The model under review builds one solid part; all positions refer to its coordinate system, in mm. A direction names the side the tool comes from. Round coordinates to 2 decimals unless told otherwise and drop trailing zeros. Write each loop counter-clockwise with the first axis right and the second up, starting at its lowest first coordinate (ties: lowest second). Pieces come first, ordered by that corner, then holes. Notation, with made-up numbers: (5, 50.5) - (31, 50.5) arc R24 ccw to (31, 76.5) - close; hole circle Ø6 at (78.5, -32.5). An arc over 180 degrees is marked (long way). Return JSON: item names as keys, results as strings.
from build123d import *

# Parameters (mm, degrees)
ESBO_O7_W                = 40
ESBO_O7_H                = 35
CORTE_EXTRUS_O3_DEPTH    = 20
ESBO_O8_W                = 40
ESBO_O8_H                = 35
RESSALTO_EXTRUS_O1_DEPTH = 60
ESBO_O9_R                = 15
CORTE_EXTRUS_O4_DEPTH    = 30
ESBO_O10_W               = 60
ESBO_O10_H               = 42.668623852
CORTE_EXTRUS_O6_DEPTH    = 5
ESBO_O12_W               = 50
ESBO_O12_H               = 21.334311926
RESSALTO_EXTRUS_O3_DEPTH = 5
ESBO_O13_W               = 60
ESBO_O13_H               = 42.668623852
CORTE_EXTRUS_O8_DEPTH    = 5
ESBO_O14_W               = 50
ESBO_O14_H               = 21.334311926
RESSALTO_EXTRUS_O4_DEPTH = 5
ESBO_O15_W               = 17.17613937
ESBO_O15_H               = 45.233285306
CORTE_EXTRUS_O9_DEPTH    = 5
ESBO_O16_W               = 17.17613937
ESBO_O16_H               = 40
RESSALTO_EXTRUS_O5_DEPTH = 5
ESBO_O17_R               = 2.5
CORTE_EXTRUS_O10_DEPTH   = 10
ESBO_O21_R               = 2.5
CORTE_EXTRUS_O11_DEPTH   = 519.156686831


with BuildPart() as part:
    # Esbo_o2 → Loft1 section 0
    with BuildSketch(Plane.XY, mode=Mode.PRIVATE) as loft1_s0:
        with BuildLine():
            Line((-10.863095238, 0), (204.136904762, 0))
            Line((204.136904762, 0), (77.102021041, 179.616642653))
            Line((77.102021041, 179.616642653), (-10.863095238, 0))
        make_face()
    loft([Vertex(77.102021041, 179.616642653, -400), loft1_s0.sketch])

    # Esbo_o7 → Corte-extrus_o3 (cut)
    with BuildSketch(Plane(origin=(77.102021041, 179.616642653, -400), x_dir=(1, 0, 0), z_dir=(0, 0, 1))):
        Rectangle(ESBO_O7_W, ESBO_O7_H)
    extrude(amount=CORTE_EXTRUS_O3_DEPTH, mode=Mode.SUBTRACT)

    # Esbo_o8 → Ressalto-extrus_o1 (add)
    with BuildSketch(Plane(origin=(0, 0, -380), x_dir=(-1, 0, 0), z_dir=(0, 0, -1))):
        with Locations((-77.5, 174.5)):
            Rectangle(ESBO_O8_W, ESBO_O8_H)
    extrude(amount=RESSALTO_EXTRUS_O1_DEPTH)

    # Esbo_o9 → Corte-extrus_o4 (cut)
    with BuildSketch(Plane(origin=(0, 192, 0), x_dir=(1, 0, 0), z_dir=(0, 1, 0))):
        with Locations(Location((77.5, 410, 0), (0, 0, 270))):
            Circle(ESBO_O9_R)
    extrude(amount=-CORTE_EXTRUS_O4_DEPTH, mode=Mode.SUBTRACT)

    # Esbo_o10 → Corte-extrus_o6 (cut)
    with BuildSketch(Plane.XY):
        with Locations((-10.863095238, 0)):
            Rectangle(ESBO_O10_W, ESBO_O10_H)
    extrude(amount=-CORTE_EXTRUS_O6_DEPTH, mode=Mode.SUBTRACT)

    # Esbo_o12 → Ressalto-extrus_o3 (add)
    with BuildSketch(Plane.XY.offset(-5)):
        with Locations((-5.863095238, 10.667155963)):
            Rectangle(ESBO_O12_W, ESBO_O12_H)
    extrude(amount=RESSALTO_EXTRUS_O3_DEPTH)

    # Esbo_o13 → Corte-extrus_o8 (cut)
    with BuildSketch(Plane.XY):
        with Locations((204.136904762, 0)):
            Rectangle(ESBO_O13_W, ESBO_O13_H)
    extrude(amount=-CORTE_EXTRUS_O8_DEPTH, mode=Mode.SUBTRACT)

    # Esbo_o14 → Ressalto-extrus_o4 (add)
    with BuildSketch(Plane.XY.offset(-5)):
        with Locations((199.136904762, 10.667155963)):
            Rectangle(ESBO_O14_W, ESBO_O14_H)
    extrude(amount=RESSALTO_EXTRUS_O4_DEPTH)

    # Esbo_o15 → Corte-extrus_o9 (cut)
    with BuildSketch(Plane.XY):
        with Locations((77.102021041, 179.616642653)):
            Rectangle(ESBO_O15_W, ESBO_O15_H)
    extrude(amount=-CORTE_EXTRUS_O9_DEPTH, mode=Mode.SUBTRACT)

    # Esbo_o16 → Ressalto-extrus_o5 (add)
    with BuildSketch(Plane.XY.offset(-5)):
        with Locations((77.102021041, 177)):
            Rectangle(ESBO_O16_W, ESBO_O16_H)
    extrude(amount=RESSALTO_EXTRUS_O5_DEPTH)

    # Esbo_o17 → Corte-extrus_o10 (cut)
    with BuildSketch(Plane.XY):
        with Locations((-20.863095238, 11.334311926)):
            Circle(ESBO_O17_R)
        with Locations((214.136904762, 10)):
            Circle(ESBO_O17_R)
        with Locations((77.190090726, 187)):
            Circle(ESBO_O17_R)
    extrude(amount=-CORTE_EXTRUS_O10_DEPTH, mode=Mode.SUBTRACT)

    # Esbo_o20 → Loft de corte2 section 0
    with BuildSketch(Plane.XY, mode=Mode.PRIVATE) as loft_de_corte2_s0:
        with BuildLine():
            Line((4.64946483, 2.5), (184.871981239, 2.5))
            Line((184.871981239, 2.5), (184.871981239, 22.909462338))
            Line((184.871981239, 22.909462338), (88.571698608, 159.069963659))
            Line((88.571698608, 159.069963659), (69.823235581, 159.069963659))
            Line((69.823235581, 159.069963659), (4.64946483, 25.99114348))
            Line((4.64946483, 25.99114348), (4.64946483, 2.5))
        make_face()
    loft([loft_de_corte2_s0.sketch, Vertex(77.102021041, 179.616642653, -400)], mode=Mode.SUBTRACT)

    # Esbo_o21 → Corte-extrus_o11 (cut, through all)
    with BuildSketch(Plane.XZ.offset(-157)):
        with Locations(Location((77.5, -410, 0), (0, 0, 270))):
            Circle(ESBO_O21_R)
    extrude(amount=-CORTE_EXTRUS_O11_DEPTH, mode=Mode.SUBTRACT)


solid = part.part
(1) For faces 1 (the flat face through (91, 192, -403)), 2 (the flat face through (143, 84, 0)), 3 (the flat face through (29.994, 71.049, -139.923)), 4 (the cylindrical face through (71.755, 177.21, -396.144)), list the 3-axis set-ups (+Z, -Z, +X, -X, +Y, -Y) from which the entire face can be reached by the end or side of a thin tool; tool diameter is ignored.
Filled in:
{"face 1": "-Z, +X, -X, +Y", "face 2": "+Z, +X, -X, +Y, -Y", "face 3": "none", "face 4": "+Y"}
(2) Wall thickness on line 1 (X direction, y = 158.55, z = -410); line 2 (X direction, y = 140.5, z = -188); line 3 (Y direction, x = 72, z = -148): over which ranges is each line inside the solid? List them lowest first.
Filled in:
{"line 1": "x = 57.5 to 75, 80 to 97.5", "line 2": "x = 57.95 to 59.42, 103.14 to 104.77", "line 3": "y = 66.46 to 68.03, 165.62 to 169.2"}
(3) Add section C-C (x = 104.5). Write out the cut boundary in (y, z), plus the area to 3 significant figures.
Filled in:
{"outline": "(0, 0) - (140.88, -313.73) - (140.88, 0) - (136.55, 0) - (139.78, -298.31) - (134.59, -298.31) - (2.5, 0) - close", "area": "1,330 mm2"}
(4) Clearance check with flat-ended pins moving along their axes: pin 1 Ø12 at (x, z) = (115.5, -72) entering from +Y; pin 2 Ø2 at (y, z) = (101, -204.5) entering from +X; pin 3 Ø10.5 at (y, z) = (168, -411.5) entering from -X. State where each tip first meets the part, or that it passes through.
Filled in:
{"pin 1": "stops at y = 133.81", "pin 2": "stops at x = 133.41", "pin 3": "stops at x = 57.5"}
(5) Add section A-A (z = -94). Write out the cut boundary in (x, y).
Filled in:
{"outline": "(9.81, 42.21) - (174.28, 42.21) - (77.1, 179.62) - close; hole (21.68, 44.12) - (159.55, 44.12) - (159.55, 59.74) - (85.88, 163.9) - (71.53, 163.9) - (21.68, 62.09) - close"}
(6) Mouldability with a two-part tool opening along X and no side actions: class faces 5 (the flat face through (97.5, 174, -410)), 6 (the flat face through (82, 157, -410)), 7 (the flat face through (74, 162, -410)) as released by +X, released by -X, zero draft, split by the parting line, or undercut.
Filled in:
{"face 5": "released by +X", "face 6": "zero draft", "face 7": "undercut"}
(7) Add section B-B (y = 86). Write out the cut boundary in (x, z), plus the area to 3 significant figures.
Filled in:
{"outline": "(31.25, -191.52) - (143.31, -191.52) - (143.31, 0) - (140.25, 0) - (141.48, -161.04) - (134.06, -188.58) - (38.81, -188.58) - (32.95, -156.25) - (34.04, 0) - (31.25, 0) - close", "area": "1,380 mm2"}
